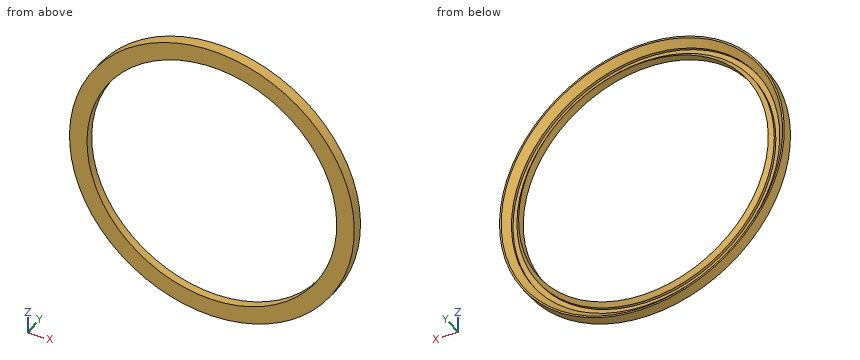
from build123d import *

# Parameters (mm, degrees)
SKETCH1_W = 5
SKETCH1_H = 5


with BuildPart() as part:
    # Sketch1 → Revolve1 (revolve)
    with BuildSketch(Plane.XY, mode=Mode.PRIVATE) as revolve1_sk:
        with Locations((30, 0)):
            Rectangle(SKETCH1_W, SKETCH1_H)
        Polygon((29.375, -1.496320344), (27.878679656, 0), (29.375, 1.496320344), (29.375, 2.121320344), (30.625, 2.121320344), (30.625, 1.496320344), (32.121320344, 0), (30.625, -1.496320344), (30.625, -2.121320344), (29.375, -2.121320344), align=None, mode=Mode.SUBTRACT)
    revolve(revolve1_sk.sketch.rotate(Axis((0, -28.665734922, 0), (0, 1, 0)), 90), axis=Axis((0, -28.665734922, 0), (0, 1, 0)))

    # Sketch2 → Cut-Revolve1 (revolve, cut)
    with BuildSketch(Plane.XY, mode=Mode.PRIVATE) as cut_revolve1_sk:
        Polygon((28.5, 0), (32.5, 0), (32.5, 2.5), (27.5, 2.5), (27.5, 0), (27.5, -2.5), (28.5, -2.5), align=None)
    revolve(cut_revolve1_sk.sketch.rotate(Axis((0, 0, 0), (0, 1, 0)), 90), axis=Axis((0, 0, 0), (0, 1, 0)), mode=Mode.SUBTRACT)


solid = part.part
The model under review builds one solid part; all positions refer to its coordinate system, in mm. Give positions to 0.01 mm unless a question says otherwise; leave off trailing zeros. Loops run counter-clockwise (first coordinate to the right, second up) from the corner with the lowest first, then second, coordinate; pieces in that order, holes last. Notation, with made-up numbers: (51.5, 34.25) -> (73.5, 34.25) arc R18 cw to (73.5, 43.25) -> close; hole circle Ø7 at (3.25, -12.75). An arc over 180 degrees is marked (long way). Put each result on its own line as item: value. Start each with the question number.
1. We need section B-B on x = 0. State the section outline as (y, z) points (3 decimals), then the cut area to 3 significant figures.
2. Clearance check with a flat-ended pin moving along its axis: P1, Ø1, axis at y = -0.5, z = 20.5, coming from the +X side. State where the tip first meets the part, or that it passes through.
3. We need section A-A on z = 0. State the section outline as (x, y) points (3 decimals).
4. We need section C-C on y = -1.1. State the section outline as (x, z) points, then the cut area to 3 significant figures.
5. Wall thickness on probe 1 along X at (y, z) = (-1.8, 0) (3 decimals); probe 2 along X at (y, z) = (-1.8, 7.5); probe 3 along Z at (x, y) = (-15, -1.8): over which ranges is each line inside the solid? List them lowest first.
Determined:
1. outline: (-2.5, -32.5) -> (0, -32.5) -> (0, -32.121) -> (-1.496, -30.625) -> (-2.121, -30.625) -> (-2.121, -29.375) -> (-1.496, -29.375) -> (-0.621, -28.5) -> (-2.5, -28.5) -> close; (-2.5, 28.5) -> (-0.621, 28.5) -> (-1.496, 29.375) -> (-2.121, 29.375) -> (-2.121, 30.625) -> (-1.496, 30.625) -> (0, 32.121) -> (0, 32.5) -> (-2.5, 32.5) -> close
1. area: 10.6 mm^2
2. P1: x = 25.62
3. outline: (-32.5, -2.5) -> (-28.5, -2.5) -> (-28.5, -0.621) -> (-29.375, -1.496) -> (-29.375, -2.121) -> (-30.625, -2.121) -> (-30.625, -1.496) -> (-32.121, 0) -> (-32.5, 0) -> close; (28.5, -2.5) -> (32.5, -2.5) -> (32.5, 0) -> (32.121, 0) -> (30.625, -1.496) -> (30.625, -2.121) -> (29.375, -2.121) -> (29.375, -1.496) -> (28.5, -0.621) -> close
4. outline: circle Ø65 at (0, 0); circle Ø57.96 at (0, 0); hole circle Ø62.04 at (0, 0); hole circle Ø57 at (0, 0)
4. area: 382 mm^2
5. probe 1: -32.5 to -30.625, -29.375 to -28.5, 28.5 to 29.375, 30.625 to 32.5
5. probe 2: -31.62 to -29.69, -28.4 to -27.5, 27.5 to 28.4, 29.69 to 31.62
5. probe 3: -28.83 to -26.7, -25.26 to -24.23, 24.23 to 25.26, 26.7 to 28.83
